from build123d import *

# Parameters (mm, degrees)
SKETCH2_W           = 85
SKETCH2_H           = 11.5
BOSS_EXTRUDE1_DEPTH = 15
SKETCH3_R           = 2.75
CUT_EXTRUDE1_DEPTH  = 10
BOSS_EXTRUDE2_DEPTH = 26
SKETCH5_R           = 2
CUT_EXTRUDE2_DEPTH  = 5


with BuildPart() as part:
    # Sketch2 → Boss-Extrude1 (new body)
    with BuildSketch(Plane(origin=(0, 0, 0), x_dir=(1, 0, 0), z_dir=(0, 1, 0))):
        Rectangle(SKETCH2_W, SKETCH2_H)
    extrude(amount=BOSS_EXTRUDE1_DEPTH)

    # Sketch3 → Cut-Extrude1 (cut)
    with BuildSketch(Plane.XZ):
        with Locations(Location((0, 0, 0), (0, 0, 270))):
            Circle(SKETCH3_R)
    extrude(amount=-CUT_EXTRUDE1_DEPTH, mode=Mode.SUBTRACT)

    # Sketch4 → Boss-Extrude2 (add)
    with BuildSketch(Plane(origin=(0, 15, 0), x_dir=(1, 0, 0), z_dir=(0, 1, 0))):
        Polygon((-42.5, 5.75), (-17.5, 5.75), (-17.5, 0.75), (-37.5, 0.75), (-37.5, -0.75), (-17.5, -0.75), (-17.5, -5.75), (-42.5, -5.75), align=None)
        Polygon((42.5, 5.75), (42.5, -5.75), (17.5, -5.75), (17.5, -0.75), (37.5, -0.75), (37.5, 0.75), (17.5, 0.75), (17.5, 5.75), align=None)
    extrude(amount=BOSS_EXTRUDE2_DEPTH)

    # Sketch5 → Cut-Extrude2 (cut)
    with BuildSketch(Plane.XY.offset(5.75)):
        with Locations((-27.5, 28.5)):
            Circle(SKETCH5_R)
        with Locations((27.5, 28.5)):
            Circle(SKETCH5_R)
    extrude(amount=-CUT_EXTRUDE2_DEPTH, mode=Mode.SUBTRACT)


solid = part.part
The listing builds one solid part. Answer for the finished solid, in the listing's coordinates (mm). A direction names the side the tool comes from. Give positions to 0.01 mm unless a question says otherwise; leave off trailing zeros. Write each loop counter-clockwise with the first axis right and the second up, starting at its lowest first coordinate (ties: lowest second). Pieces come first, ordered by that corner, then holes. Notation, with made-up numbers: (-18.5, 74) - (-12.5, 74) arc R16 ccw to (-12.5, 98) - close; hole circle Ø7 at (-11, -33). An arc over 180 degrees is marked (long way). One line per question, with ' | ' between items. Start each with the question number.
1. Section D-D, the plane y = 35 is taken. Determine the outline of the cut face in (x, z).
2. Given P1, Ø5, axis at x = 0, z = 0, coming from the +Y side, flat-ended and moving along its own axis, determine where the tip first touches the part or whether it passes through.
3. Straight lines are drawn through the part: line 1 (Y direction, x = -27.5, z = 2.65); line 2 (X direction, y = 29.5, z = 1.5); line 3 (Z direction, x = -26, y = 23). For each, find the intervals that lie inside material, in ascending order.
4. For faces 5 (the face through (1, 11, 5.75)), 6 (the face through (17.5, 28, -3)), 7 (the face through (-27, 28, -0.75)), 8 (the face through (0, 10, 0)), determine the directions among +Z, -Z, +X, -X, +Y, -Y from which every point of the face is accessible in a straight line to the end or side of a thin tool.
5. Section B-B, the plane y = 28.5 is taken. Determine the outline of the cut face in (x, z).
6. Section A-A, the plane x = 27.5 is taken. Determine the outline of the cut face in (y, z), then the cut area to 4 significant figures.
7. Determine the mould class of faces 1 (the face through (-17.5, 28, 3)), 2 (the face through (-26.577, 26.726, 3.285)), 3 (the face through (28.423, 26.726, 3.285)), 4 (the face through (-1, 0, 4)) for opening direction Y: +Y half, -Y half, draft (parallel to the pull), parting line (faces both ways), or undercut.
8. Section C-C, the plane z = 4.25 is taken. Determine the outline of the cut face in (x, y).
Result:
1) outline: (-42.5, -5.75) - (-17.5, -5.75) - (-17.5, -0.75) - (-37.5, -0.75) - (-37.5, 0.75) - (-17.5, 0.75) - (-17.5, 5.75) - (-42.5, 5.75) - close; (17.5, -5.75) - (42.5, -5.75) - (42.5, 5.75) - (17.5, 5.75) - (17.5, 0.75) - (37.5, 0.75) - (37.5, -0.75) - (17.5, -0.75) - close
2) P1: stops at y = 15
3) line 1: y = 0 to 26.5, 30.5 to 41 | line 2: x = -42.5 to -29.23, -25.77 to -17.5, 17.5 to 25.77, 29.23 to 42.5 | line 3: z = -5.75 to -0.75, 0.75 to 5.75
4) face 5: +Z, +X, -X, +Y, -Y | face 6: +Z, -Z, +Y | face 7: +Y | face 8: -Y
5) outline: (-42.5, -5.75) - (-17.5, -5.75) - (-17.5, -0.75) - (-37.5, -0.75) - (-37.5, 0.75) - (-29.5, 0.75) - (-29.5, 5.75) - (-42.5, 5.75) - close; (-25.5, 0.75) - (-17.5, 0.75) - (-17.5, 5.75) - (-25.5, 5.75) - close; (17.5, -5.75) - (42.5, -5.75) - (42.5, 5.75) - (29.5, 5.75) - (29.5, 0.75) - (37.5, 0.75) - (37.5, -0.75) - (17.5, -0.75) - close; (17.5, 0.75) - (25.5, 0.75) - (25.5, 5.75) - (17.5, 5.75) - close
6) outline: (0, -5.75) - (41, -5.75) - (41, -0.75) - (15, -0.75) - (15, 0.75) - (26.5, 0.75) - (26.5, 5.75) - (0, 5.75) - close; (30.5, 0.75) - (41, 0.75) - (41, 5.75) - (30.5, 5.75) - close | area: 412.5 mm2
7) face 1: draft | face 2: undercut | face 3: undercut | face 4: -Y half
8) outline: (-42.5, 0) - (42.5, 0) - (42.5, 41) - (17.5, 41) - (17.5, 15) - (-17.5, 15) - (-17.5, 41) - (-42.5, 41) - close; hole circle Ø4 at (-27.5, 28.5); hole circle Ø4 at (27.5, 28.5)
